```python
from build123d import *

# Parameters (mm, degrees)
SALIENTE_EXTRUIR1_DEPTH = 76.2
CROQUIS4_R              = 3.81
CORTAR_EXTRUIR1_DEPTH   = 2.54
CORTAR_EXTRUIR1_TAPER   = 39
CROQUIS5_R              = 3.81
CORTAR_EXTRUIR2_DEPTH   = 2.54
CORTAR_EXTRUIR2_TAPER   = 39


with BuildPart() as part:
    # Croquis1 → Saliente-Extruir1 (new body)
    with BuildSketch(Plane(origin=(0, 0, 0), x_dir=(0, 0, -1), z_dir=(1, 0, 0))):
        with BuildLine():
            Line((-40.64, -351.79000001), (-86.135923686, 93.325251946))
            ThreePointArc((-86.135923686, 93.325251946), (0, 127), (86.135923686, 93.325251946))
            Line((86.135923686, 93.325251946), (40.64, -351.79000001))
            Line((40.64, -351.79000001), (-40.64, -351.79000001))
        make_face()
    extrude(amount=SALIENTE_EXTRUIR1_DEPTH)

    # Croquis4 → Cortar-Extruir1 (cut)
    with BuildSketch(Plane(origin=(76.2, 0, 0), x_dir=(0, 0, -1), z_dir=(1, 0, 0))):
        with Locations((-49.917099877, -136.126844727)):
            Circle(CROQUIS4_R)
        with Locations((-38.362373799, -249.174001321)):
            Circle(CROQUIS4_R)
        with Locations((-34.768096531, -284.339077712)):
            Circle(CROQUIS4_R)
        with Locations((-29.171919425, -339.09000001)):
            Circle(CROQUIS4_R)
        with Locations((29.171919425, -339.09000001)):
            Circle(CROQUIS4_R)
        with Locations((4.819460737, -284.339077712)):
            Circle(CROQUIS4_R)
    extrude(amount=-CORTAR_EXTRUIR1_DEPTH, taper=CORTAR_EXTRUIR1_TAPER, mode=Mode.SUBTRACT)

    # Croquis5 → Cortar-Extruir2 (cut)
    with BuildSketch(Plane.ZY):
        with Locations((-12.556850651, -339.09000001)):
            Circle(CROQUIS5_R)
        with Locations((12.556850651, -339.09000001)):
            Circle(CROQUIS5_R)
        with Locations((-34.182100121, -290.072249352)):
            Circle(CROQUIS5_R)
        with Locations((-48.265473167, -152.285748198)):
            Circle(CROQUIS5_R)
        with Locations((-69.751939629, 57.929874619)):
            Circle(CROQUIS5_R)
        with Locations((-48.265473167, 103.609527072)):
            Circle(CROQUIS5_R)
        with Locations((48.265473167, 103.609527072)):
            Circle(CROQUIS5_R)
        with Locations((69.751939629, 57.929874619)):
            Circle(CROQUIS5_R)
        with Locations((48.265473167, -152.285748198)):
            Circle(CROQUIS5_R)
    extrude(amount=-CORTAR_EXTRUIR2_DEPTH, taper=CORTAR_EXTRUIR2_TAPER, mode=Mode.SUBTRACT)


solid = part.part
```
Can you work these out from the model? Positions are in its coordinate system, mm. Give positions to 0.01 mm unless a question says otherwise; leave off trailing zeros. Order: outer loops, then holes, each group sorted by start corner. A loop starts at its lowest first (then second) coordinate and runs counter-clockwise, first axis right, second up. Notation, with made-up numbers: (5.5, -5) - (51.5, -5) arc R32 cw to (51.5, 33) - close; hole circle Ø10 at (65.25, 30). An arc over 180 degrees is marked (long way). Use a Markdown table: item, result. Add a question column.
Q1. If we section it at B-B on y = -39.5: Write out the boundary of the cut face in (x, z), plus the area to 3 significant figures.
Q2. Please list where these lines run through material, in increasing order: line 1 along Y through (x, z) = (33.5, 2); line 2 along Y through (x, z) = (31, 33.5); line 3 along Z through (x, y) = (54.5, -32.5).
Q3. If we section it at A-A on x = 49: Write out the boundary of the cut face in (y, z), plus the area to 3 significant figures.
Q4. I'm going to push flat-ended pins straight in: pin 1 (3 mm diameter, centred on y = 58.5, z = 70, fed in from -X); pin 2 (1.5 mm diameter, centred on x = 19, y = -265.5, fed in from -Z); pin 3 (6 mm diameter, centred on x = 57, y = -86.5, fed in from +Z). Where does each tip first touch, or does it pass through?
Answers follow:
| question | item | result |
|---|---|---|
| 1 | outline | (0, -72.56) - (76.2, -72.56) - (76.2, 72.56) - (0, 72.56) - close |
| 1 | area | 11,100 mm^2 |
| 2 | line 1 | y = -351.79 to 126.98 |
| 2 | line 2 | y = -351.79 to 122.5 |
| 2 | line 3 | z = -73.28 to 73.28 |
| 3 | outline | (-351.79, -40.64) - (93.33, -86.14) arc R127 ccw to (93.33, 86.14) - (-351.79, 40.64) - close |
| 3 | area | 60,400 mm^2 |
| 4 | pin 1 | stops at x = 2.08 |
| 4 | pin 2 | stops at z = -49.54 |
| 4 | pin 3 | stops at z = 68.06 |
